Can you work these out from the model? Positions are in its coordinate system, mm. A direction names the side the tool comes from. Give positions to 0.01 mm unless a question says otherwise; leave off trailing zeros. Loops run counter-clockwise (first coordinate to the right, second up) from the corner with the lowest first, then second, coordinate; pieces in that order, holes last. Notation, with made-up numbers: M 50.25,-4.5 L 94.25,-4.5 A15 ccw 94.25,17.5 Z; hole C 85,-11 d5. An arc over 180 degrees is marked long. One line per item, written item: value. Start each with the question number.
from build123d import *

# Parameters (mm, degrees)
F2_W          = 304.8
F2_H          = 304.8
F3_DEPTH      = 6.35
F5_R          = 36.5125
F5_R_2        = 30.1625
F6_DEPTH      = 292.1
F6_DEPTH_BACK = 12.7
F8_DEPTH      = 50.8
F8_DEPTH_BACK = 50.8
F9_R          = 4.7625
F10_DEPTH     = 2.54
F11_R         = 6.35
F12_DEPTH     = 25.4


with BuildPart() as f3:
    # F2 (on line) → F3 (new body)
    with BuildSketch(Plane(origin=(0, 0, 0), x_dir=(1, 0, 0), z_dir=(0, 0.1736481777, 0.984807753))):
        Rectangle(F2_W, F2_H)
    extrude(amount=F3_DEPTH)

    # F5 (on line) → F6 (join, two sides)
    with BuildSketch(Plane(origin=(6.35, 0, -10.9985226281), x_dir=(0.8660254038, 0, 0.5), z_dir=(0.5, 0, -0.8660254038))) as f6_sk:
        Circle(F5_R)
        Circle(F5_R_2, mode=Mode.SUBTRACT)
    extrude(amount=-F6_DEPTH)
    extrude(f6_sk.sketch, amount=F6_DEPTH_BACK)

    # F7 (on Right) → F8 (cut, two sides)
    with BuildSketch(Plane.YZ) as f8_sk:
        Polygon((56.8870845878, -43.9009879504), (56.8870845878, -10.0307278667), (-39.12624161, 6.8990120496), (-39.12624161, -43.9009879504), align=None)
    extrude(amount=-F8_DEPTH, mode=Mode.SUBTRACT)
    extrude(f8_sk.sketch, amount=F8_DEPTH_BACK, mode=Mode.SUBTRACT)

    # F9 (on face) → F10 (cut)
    with BuildSketch(Plane(origin=(0, 1.1026659282, 6.2535292316), x_dir=(1, 0, 0), z_dir=(0, 0.1736481777, 0.984807753))):
        with Locations((0, -76.2)):
            Circle(F9_R)
        with Locations((0, -127)):
            Circle(F9_R)
        with Locations((-127, 0)):
            Circle(F9_R)
        with Locations((-76.2, 0)):
            Circle(F9_R)
    extrude(amount=-F10_DEPTH, mode=Mode.SUBTRACT)

    # F11 (on face) → F12 (cut)
    with BuildSketch(Plane(origin=(0, 1.1026659282, 6.2535292316), x_dir=(1, 0, 0), z_dir=(0, 0.1736481777, 0.984807753))):
        with Locations((127, 127)):
            Circle(F11_R)
        with Locations((127, -127)):
            Circle(F11_R)
        with Locations((-127, -127)):
            Circle(F11_R)
        with Locations((-127, 127)):
            Circle(F11_R)
    extrude(amount=-F12_DEPTH, mode=Mode.SUBTRACT)


solid = f3.part
Q1. I need wall thicknesses on line 1 along Y through (x, z) = (-53.5, 142); line 2 along Z through (x, y) = (-32.5, 7.5); line 3 along X through (y, z) = (22, 227.5). Which ranges of each line are inside material? Lowest first, please.
Q2. If we mould it in two halves opening along Z, with no side actions, what happens to faces 1 (the face through (133.057, 127.508, -19.214)), 2 (the face through (152.4, -2, 3)), 3 (the face through (2.198, -128.346, 27.807))? For each: released by +Z, released by -Z, zero draft, split by the parting line, or undercut.
Q3. If we section it at B-B, the plane y = 113: Write out the boundary of the cut face in (x, z).
Q4. For P1, Ø10, axis at y = -4, z = 203.5, coming from the +X side; P2, Ø10, axis at x = -107, y = 103, coming from the +Z side; P3, Ø2, axis at x = -114, y = -19, coming from the +Z side, each with a flat end and sliding along its axis, tell me the tip position at first contact or that it passes through.
Q5. If we section it at A-A, the plane x = -92: Give the number of separate pieces and of enclosed holes in the cut face, plus the area to 3 significant figures.
Q6. Which directions (+Z, -Z, +X, -X, +Y, -Y) give clear straight access to the entire face, cutting with the end or side of a thin tool? Please do faces 4 (the face through (-152.4, -2, 3)), 5 (the face through (-135.16, -29.92, 244.59)), 6 (the face through (-76.27, 0.73, 3.74)).
Response:
1. line 1: -26.92 to -17.36, 17.36 to 26.92
1. line 2: -1.32 to 5.13, 114.72 to 127.76
1. line 3: -164.76 to -155.17, -107.52 to -97.7
2. face 1: split by the parting line
2. face 2: zero draft
2. face 3: undercut
3. outline: M -152.4,-19.92 L 152.4,-19.92 L 152.4,-13.48 L -152.4,-13.48 Z
4. P1: x = -72.64
4. P2: z = -10.83
4. P3: z = 257.38
5. separate pieces: 2
5. enclosed holes: 1
5. area: 4,600 mm^2
6. face 4: -Z, -X, +Y, -Y
6. face 5: +Z, -X, +Y, -Y
6. face 6: none
